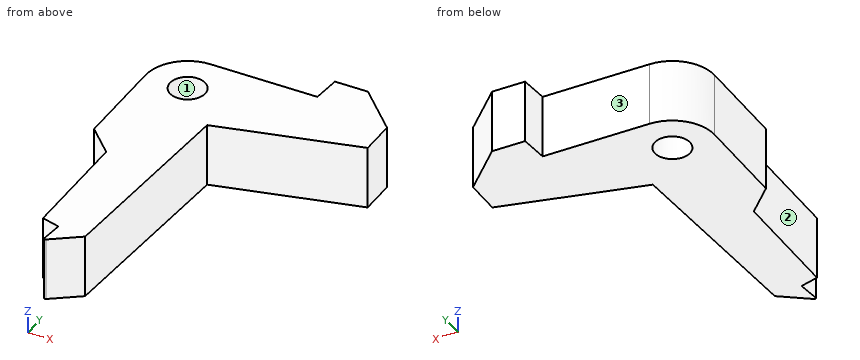
```python
from build123d import *

# Parameters (mm, degrees)
SKETCH_1_R      = 6
SKETCH_1_R_2    = 2.5
EXTRUDE_1_DEPTH = 9


with BuildPart() as part:
    # 스케치1 → 보스-돌출1 (new body)
    # profile 1 of 2: a face of its own
    with BuildSketch(Plane.XY):
        with BuildLine():
            Line((15.138175611, 6), (0, 6))
            ThreePointArc((0, 6), (4.242640687, 4.242640687), (6, 0))
            ThreePointArc((6, 0), (0, -6), (-6, 0))
            Line((-6, 0), (-6, -13.433276283))
            Line((-6, -13.433276283), (-2.272089827, -17.161186456))
            Line((-2.272089827, -17.161186456), (-2.272089827, -33.747703831))
            Line((-2.272089827, -33.747703831), (0.282693742, -34.440633794))
            Line((0.282693742, -34.440633794), (-0.033215199, -37.525789008))
            ThreePointArc((-0.033215199, -37.525789008), (0.065651627, -37.719313216), (0.282693742, -37.70840501))
            Line((0.282693742, -37.70840501), (4.278390118, -34.828200083))
            Line((4.278390118, -34.828200083), (6, -6))
            Line((6, -6), (25.995290484, -0.925171702))
            Line((25.995290484, -0.925171702), (25.995290484, 4.149656597))
            Line((25.995290484, 4.149656597), (20.144947081, 10))
            Line((20.144947081, 10), (15.462448132, 10))
            Line((15.462448132, 10), (15.138175611, 6))
        make_face()
    # profile 2 of 2: a face of its own
    with BuildSketch(Plane.XY):
        Circle(SKETCH_1_R)
        Circle(SKETCH_1_R_2, mode=Mode.SUBTRACT)
    extrude(amount=EXTRUDE_1_DEPTH)


solid = part.part
```
Source: CAD feature listing. Evaluate the final solid. Frame: model axes, mm. Face numbers are marked on the shaded views. Give positions to 0.01 mm unless a question says otherwise; leave off trailing zeros. Loops run counter-clockwise (first coordinate to the right, second up) from the corner with the lowest first, then second, coordinate; pieces in that order, holes last. Notation, with made-up numbers: (-10, 21) -> (-5, 21) arc R12 cw to (-5, 39) -> close; hole circle Ø7 at (-15, 45). An arc over 180 degrees is marked (long way). Put each result on its own line as item: value. Start each with the question number.
1) Contact query for flat-ended pins moving along their axis: P1, Ø4, axis at x = 0, y = 0, coming from the -Z side; P2, Ø1, axis at y = -14.5, z = 2.5, coming from the +X side; P3, Ø2.5, axis at x = 4.5, z = 3, coming from the +Y side; P4, Ø1.5, axis at x = -1, z = 6, coming from the -Y side. Output: stop coordinate, or through.
2) Cut plane B-B (x = -0.5). Return loops of the section in (y, z).
3) Draft query along X for the marked faces 1, 2 and 3. Return one class per face: released by +X, released by -X, zero draft, split by the parting line, or undercut.
4) Cut plane D-D (x = 10). Return loops of the section in (y, z).
5) Material intervals for probe 1 along X at (y, z) = (-13.5, 4); probe 2 along Y at (x, z) = (-1, 7.25); probe 3 along X at (y, z) = (-15.5, 8.75), sorted ascending.
6) Cut plane C-C (y = -4). Return loops of the section in (x, z).
7) Cut plane A-A (z = 5.75). Return loops of the section in (x, y).
Results are:
1. P1: passes through
1. P2: stops at x = 5.52
1. P3: stops at y = 6
1. P4: stops at y = -34.3
2. outline: (-34.23, 0) -> (-2.45, 0) -> (-2.45, 9) -> (-34.23, 9) -> close; (2.45, 0) -> (5.98, 0) -> (5.98, 9) -> (2.45, 9) -> close
3. face 1: undercut
3. face 2: released by -X
3. face 3: zero draft
4. outline: (-4.98, 0) -> (6, 0) -> (6, 9) -> (-4.98, 9) -> close
5. probe 1: x = -5.93 to 5.55
5. probe 2: y = -34.09 to -2.29, 2.29 to 5.92
5. probe 3: x = -3.93 to 5.43
6. outline: (-6, 0) -> (13.88, 0) -> (13.88, 9) -> (-6, 9) -> close
7. outline: (-6, -13.43) -> (-2.27, -17.16) -> (-2.27, -33.75) -> (0.28, -34.44) -> (-0.03, -37.53) arc R0.2 ccw to (0.28, -37.71) -> (4.28, -34.83) -> (6, -6) -> (26, -0.93) -> (26, 4.15) -> (20.14, 10) -> (15.46, 10) -> (15.14, 6) -> (0, 6) arc R6 ccw to (-6, 0) -> close; hole circle Ø5 at (0, 0)
